```python
from build123d import *

# Parameters (mm, degrees)
SKETCH1_W           = 100.33
SKETCH1_H           = 63.5
BOSS_EXTRUDE1_DEPTH = 24.638
SKETCH3_W           = 10.16
SKETCH3_H           = 8.89
SKETCH3_W_2         = 13.97
SKETCH3_H_2         = 6.604
CUT_EXTRUDE1_DEPTH  = 25.4
SKETCH4_W           = 10.414
SKETCH4_H           = 15.24
BOSS_EXTRUDE2_DEPTH = 5.08


with BuildPart() as part:
    # Sketch1 → Boss-Extrude1 (new body)
    with BuildSketch(Plane.XY):
        Rectangle(SKETCH1_W, SKETCH1_H)
    extrude(amount=BOSS_EXTRUDE1_DEPTH)

    # Sketch3 → Cut-Extrude1 (cut)
    with BuildSketch(Plane.ZY.offset(50.165)):
        with Locations((13.97, 18.415)):
            Rectangle(SKETCH3_W, SKETCH3_H)
        with Locations((12.065, 6.604)):
            Rectangle(SKETCH3_W_2, SKETCH3_H_2)
    extrude(amount=-CUT_EXTRUDE1_DEPTH, mode=Mode.SUBTRACT)

    # Sketch4 → Boss-Extrude2 (add)
    with BuildSketch(Plane.ZY.offset(50.165)):
        with Locations((12.319, -13.97)):
            Rectangle(SKETCH4_W, SKETCH4_H)
    extrude(amount=BOSS_EXTRUDE2_DEPTH)


solid = part.part
```
Could you check a few things on this model? Use its own coordinates, in mm. A direction names the side the tool comes from. Round coordinates to 2 decimals unless told otherwise and drop trailing zeros. Write each loop counter-clockwise with the first axis right and the second up, starting at its lowest first coordinate (ties: lowest second). Pieces come first, ordered by that corner, then holes. Notation, with made-up numbers: M -36.75,-14.5 L 18.25,-14.5 A6 ccw 18.25,-4.5 Z; hole C -4.5,34 d5. An arc over 180 degrees is marked long. Write each question's results on one line, items separated by ' | '. Start each with the question number.
1. I need wall thicknesses on L1, parallel to Y at x = -44.5, z = 12.5; L2, parallel to Z at x = -43, y = 20; L3, parallel to Y at x = -49, z = 7. Which ranges of each line are inside material? Lowest first, please. Write a range as from..to.
2. Imagine slicing it at A-A on z = 11. List the corners of the cut face in (x, y) for me (3 decimals).
3. Imagine slicing it at B-B on y = 18. List the corners of the cut face in (x, z) for me (3 decimals).
4. Imagine slicing it at C-C on x = -40. List the corners of the cut face in (y, z) for me.
5. On a 3-axis mill with a long thin cutter (end or side, diameter ignored), from which of +Z, -Z, +X, -X, +Y, -Y can I reach the whole of each face in a straight line? I mean faces 1 (the face through (-24.765, 18, 14)), 2 (the face through (50.165, 0, 12)), 3 (the face through (-53, -6.35, 12)). Say none if no direction works.
6. Imagine slicing it at D-D on y = -23. List the corners of the cut face in (x, z) for me (3 decimals).
7. Thinking about a two-plate mould opening in Y: for faces 4 (the face through (-53, -21.59, 12)), 5 (the face through (-38, 3.302, 12)), 6 (the face through (-53, -14, 7.112)), which applies, +Y half, -Y half, draft (parallel to the pull), parting line (faces both ways), or undercut?
8. I'm going to push flat-ended pins straight in: pin 1 Ø8 at (y, z) = (-0.5, 8.5) entering from -X (3 decimals); pin 2 Ø2.5 at (x, z) = (-52.5, 11) entering from -Y; pin 3 Ø1.5 at (x, y) = (-53, -16) entering from -Z. Where does each tip first touch, or does it pass through?
Result sheet:
1) L1: y = -31.75..3.3, 9.91..13.97, 22.86..31.75 | L2: z = 0..8.89, 19.05..24.64 | L3: y = -31.75..3.3, 9.91..31.75
2) outline: M -55.245,-21.59 L -50.165,-21.59 L -50.165,-31.75 L 50.165,-31.75 L 50.165,31.75 L -50.165,31.75 L -50.165,22.86 L -24.765,22.86 L -24.765,13.97 L -50.165,13.97 L -50.165,9.906 L -24.765,9.906 L -24.765,3.302 L -50.165,3.302 L -50.165,-6.35 L -55.245,-6.35 Z
3) outline: M -50.165,0 L 50.165,0 L 50.165,24.638 L -50.165,24.638 L -50.165,19.05 L -24.765,19.05 L -24.765,8.89 L -50.165,8.89 Z
4) outline: M -31.75,0 L 31.75,0 L 31.75,24.64 L -31.75,24.64 Z; hole M 3.3,5.08 L 9.91,5.08 L 9.91,19.05 L 3.3,19.05 Z; hole M 13.97,8.89 L 22.86,8.89 L 22.86,19.05 L 13.97,19.05 Z
5) face 1: -X | face 2: +Z, -Z, +X, +Y, -Y | face 3: +Z, -Z, -X, +Y
6) outline: M -50.165,0 L 50.165,0 L 50.165,24.638 L -50.165,24.638 Z
7) face 4: -Y half | face 5: undercut | face 6: draft
8) pin 1: stops at x = -50.165 | pin 2: stops at y = -21.59 | pin 3: stops at z = 7.11
